The listing builds one solid part. Answer for the finished solid, in the listing's coordinates (mm). Give positions to 0.01 mm unless a question says otherwise; leave off trailing zeros. Loops run counter-clockwise (first coordinate to the right, second up) from the corner with the lowest first, then second, coordinate; pieces in that order, holes last. Notation, with made-up numbers: (-11.75, 12.5) - (15.25, 12.5) arc R26 ccw to (15.25, 49.5) - close; hole circle Ø8 at (64.25, 71.5). An arc over 180 degrees is marked (long way). One line per item, written item: value. Start each with the question number.
from build123d import *

# Parameters (mm, degrees)
BOSS_EXTRUDE1_DEPTH = 5


with BuildPart() as part:
    # Sketch1 → Boss-Extrude1 (new body)
    with BuildSketch(Plane(origin=(0, 0, 0), x_dir=(1, 0, 0), z_dir=(0, 1, 0))):
        with BuildLine():
            Line((-183.2, 108.2), (-109.92, 108.2))
            Line((-109.92, 108.2), (-109.92, 105.5))
            Line((-109.92, 105.5), (-36.64, 105.5))
            Line((-36.64, 105.5), (-36.64, 108.2))
            Line((-36.64, 108.2), (36.64, 108.2))
            Line((36.64, 108.2), (36.64, 105.5))
            Line((36.64, 105.5), (109.92, 105.5))
            Line((109.92, 105.5), (109.92, 108.2))
            Line((109.92, 108.2), (183.2, 108.2))
            Line((183.2, 108.2), (183.2, 105.5))
            Line((183.2, 105.5), (180.5, 105.5))
            Line((180.5, 105.5), (180.5, 63.3))
            Line((180.5, 63.3), (183.2, 63.3))
            Line((183.2, 63.3), (183.2, 21.1))
            Line((183.2, 21.1), (180.5, 21.1))
            Line((180.5, 21.1), (180.5, -21.1))
            Line((180.5, -21.1), (183.2, -21.1))
            Line((183.2, -21.1), (183.2, -63.3))
            Line((183.2, -63.3), (180.5, -63.3))
            Line((180.5, -63.3), (180.5, -105.5))
            Line((180.5, -105.5), (183.2, -105.5))
            Line((183.2, -105.5), (183.2, -108.2))
            Line((183.2, -108.2), (109.92, -108.2))
            Line((109.92, -108.2), (109.92, -105.5))
            Line((109.92, -105.5), (36.64, -105.5))
            Line((36.64, -105.5), (36.64, -108.2))
            Line((36.64, -108.2), (76.64, -108.2))
            Line((76.64, -108.2), (76.64, -112.2))
            Line((76.64, -112.2), (48.383969685, -116.8270792))
            ThreePointArc((48.383969685, -116.8270792), (42.378966502, -120.22108374), (40, -126.695637657))
            Line((40, -126.695637657), (40, -144.759693491))
            ThreePointArc((40, -144.759693491), (41.977070717, -150.728998787), (47.126521144, -154.337956343))
            Line((47.126521144, -154.337956343), (60, -158.2))
            Line((60, -158.2), (40, -158.2))
            Line((40, -158.2), (24, -158.2))
            Line((24, -158.2), (24, -153.2))
            Line((24, -153.2), (8, -153.2))
            Line((8, -153.2), (8, -158.2))
            Line((8, -158.2), (-8, -158.2))
            Line((-8, -158.2), (-8, -153.2))
            Line((-8, -153.2), (-24, -153.2))
            Line((-24, -153.2), (-24, -158.2))
            Line((-24, -158.2), (-40, -158.2))
            Line((-40, -158.2), (-60, -158.2))
            Line((-60, -158.2), (-47.126521144, -154.337956343))
            ThreePointArc((-47.126521144, -154.337956343), (-41.977070717, -150.728998787), (-40, -144.759693491))
            Line((-40, -144.759693491), (-40, -126.695637657))
            ThreePointArc((-40, -126.695637657), (-42.378966502, -120.22108374), (-48.383969685, -116.8270792))
            Line((-48.383969685, -116.8270792), (-76.64, -112.2))
            Line((-76.64, -112.2), (-76.64, -108.2))
            Line((-76.64, -108.2), (-36.64, -108.2))
            Line((-36.64, -108.2), (-36.64, -105.5))
            Line((-36.64, -105.5), (-109.92, -105.5))
            Line((-109.92, -105.5), (-109.92, -108.2))
            Line((-109.92, -108.2), (-183.2, -108.2))
            Line((-183.2, -108.2), (-183.2, -105.5))
            Line((-183.2, -105.5), (-180.5, -105.5))
            Line((-180.5, -105.5), (-180.5, -63.3))
            Line((-180.5, -63.3), (-183.2, -63.3))
            Line((-183.2, -63.3), (-183.2, -21.1))
            Line((-183.2, -21.1), (-180.5, -21.1))
            Line((-180.5, -21.1), (-180.5, 21.1))
            Line((-180.5, 21.1), (-183.2, 21.1))
            Line((-183.2, 21.1), (-183.2, 63.3))
            Line((-183.2, 63.3), (-180.5, 63.3))
            Line((-180.5, 63.3), (-180.5, 105.5))
            Line((-180.5, 105.5), (-183.2, 105.5))
            Line((-183.2, 105.5), (-183.2, 108.2))
        make_face()
    extrude(amount=BOSS_EXTRUDE1_DEPTH)


solid = part.part
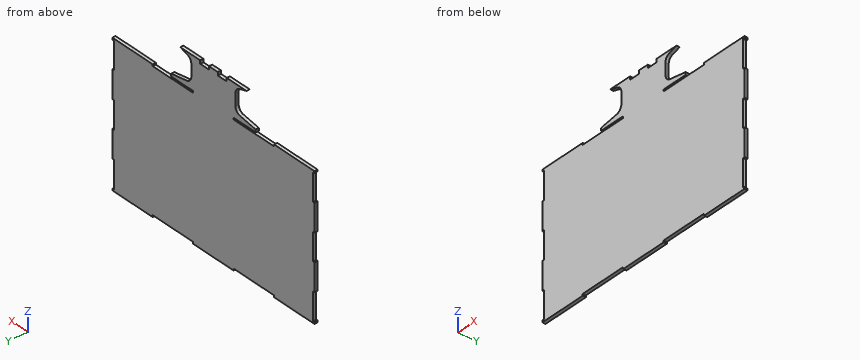
1. A cutting plane is placed at A-A (z = 131.5). Determine the outline of the cut face in (x, y).
2. A cutting plane is placed at B-B (x = 82). Determine the outline of the cut face in (y, z), plus the area to 4 significant figures.
3. Find the intervals of material crossed by L1, parallel to X at y = 4.6, z = -64; L2, parallel to Z at x = -126, y = 2.9; L3, parallel to X at y = 2.3, z = 129, in increasing order. Write a range as [from, to].
4. Flat-ended cylindrical pins translate along their axes: pin 1 (3 mm diameter, centred on x = -182.5, y = 2.5, fed in from +Z); pin 2 (1.5 mm diameter, centred on y = 1.5, z = 134, fed in from -X); pin 3 (1 mm diameter, centred on x = -71, y = 1, fed in from -Z). Find the tip coordinate at first contact, or state that the pin passes through.
Results below:
1. outline: (-40, 0) - (40, 0) - (40, 5) - (-40, 5) - close
2. outline: (0, -105.5) - (5, -105.5) - (5, 105.5) - (0, 105.5) - close
2. area: 1,055 mm^2
3. L1: x = [-180.5, 180.5]
3. L2: z = [-108.2, 108.2]
3. L3: x = [-40, 40]
4. pin 1: stops at z = 108.2
4. pin 2: stops at x = -40
4. pin 3: stops at z = -105.5
